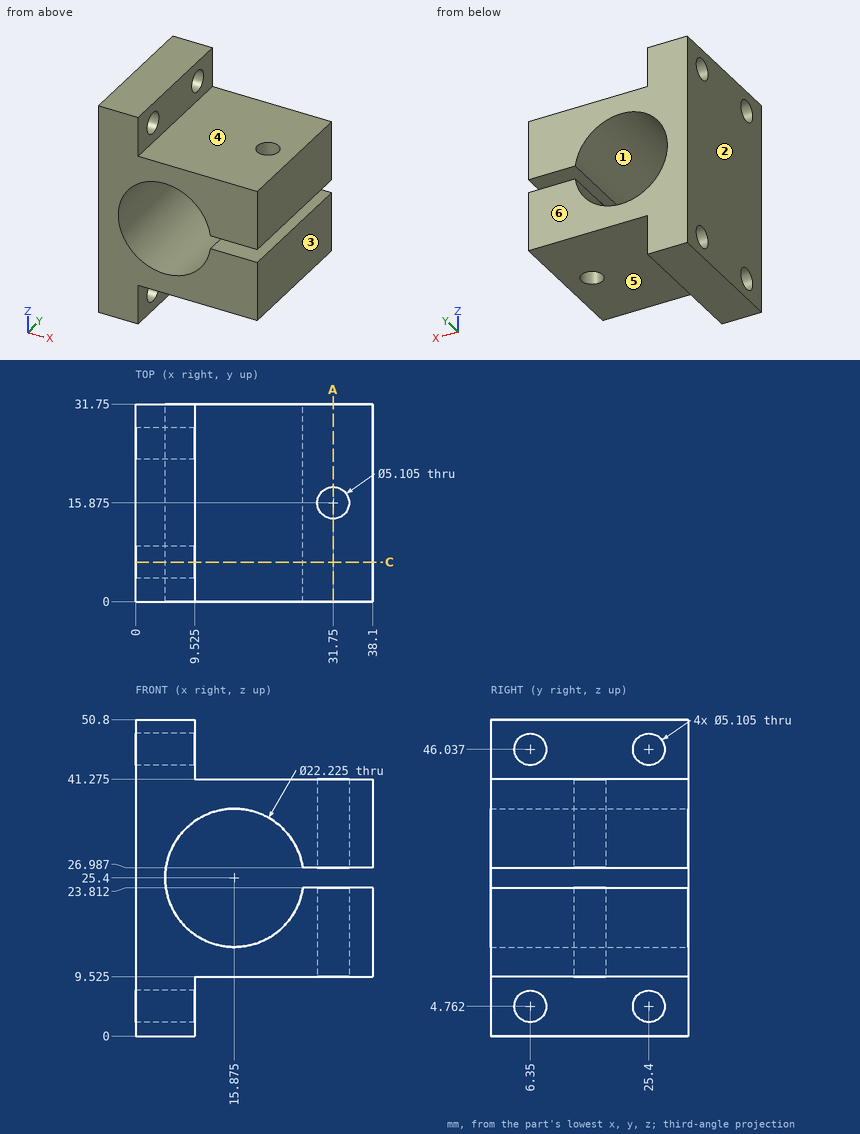
Source: three-view drawing plus pictorial views. Frame: mm from the lowest corner of the part. A direction names the side the tool comes from. Round coordinates to 2 decimals unless told otherwise and drop trailing zeros. Loops run counter-clockwise (first coordinate to the right, second up) from the corner with the lowest first, then second, coordinate; pieces in that order, holes last.
Q1. Section C-C on y = 6.35. Return loops of the section in (x, z) (1 decimal).
Q2. Section A-A on x = 31.75. State how many separate pieces and enclosed holes the cut face has.
Q3. Access query for the marked faces 4, 5 and 6. Directions: +Z, -Z, +X, -X, +Y, -Y. A direction counts if a zero-diameter tool reaches every point of the face in a straight line with its end or side. Return the directions, or none.
Q4. Pull-direction query (X, two-part tool) for the marked faces 1, 2 and 3; classes: released by +X, released by -X, zero draft, split by the parting line, or undercut.
Q5. Material intervals for L1, parallel to Y at x = 31.75, z = 17.25; L2, parallel to Z at x = 33.5, y = 21 (1 decimal); L3, parallel to X at y = 16, z = 39, sorted ascending.
Q6. Pin query (flat end, axial travel): P1, Ø4, axis at x = 26, y = 23, coming from the +Z side (1 decimal); P2, Ø5, axis at y = 22.5, z = 6.5, coming from the +X side (1 decimal); P3, Ø12.5, axis at x = 31, y = 10, coming from the -Z side (1 decimal). Return the tip coordinate at first contact, or that it passes through.
Evaluation:
1. outline: (0, 0) - (9.5, 0) - (9.5, 2.2) - (0, 2.2) - close; (0, 7.3) - (9.5, 7.3) - (9.5, 9.5) - (38.1, 9.5) - (38.1, 23.8) - (26.9, 23.8) arc R11.1 cw (long way) to (26.9, 27) - (38.1, 27) - (38.1, 41.3) - (9.5, 41.3) - (9.5, 43.5) - (0, 43.5) - close; (0, 48.6) - (9.5, 48.6) - (9.5, 50.8) - (0, 50.8) - close
2. separate pieces: 4
2. enclosed holes: 0
3. face 4: +Z, +X, +Y, -Y
3. face 5: -Z, +X, +Y, -Y
3. face 6: +Z, -Z, +X, -X, +Y
4. face 1: undercut
4. face 2: released by -X
4. face 3: released by +X
5. L1: y = 0 to 13.32, 18.43 to 31.75
5. L2: z = 9.5 to 23.8, 27 to 41.3
5. L3: x = 0 to 29.2, 34.3 to 38.1
6. P1: stops at z = 41.3
6. P2: stops at x = 9.5
6. P3: stops at z = 9.5
